Autodesk Fusion 360 part; units mm, degrees
box "BoxPrimitive5" add length 100 width 90 height 2 placed x (0, 0, -1) y (-1, 0, 0) z (0, 1, 0) at (0, 0, 0)
box "BoxPrimitive6" cut length 9 width 4 height -14 placed x (0, 0, 1) y (1, 0, 0) z (0, 1, 0) at (-6, 2, -9)
box "BoxPrimitive7" cut length 9 width 9 height -11 placed x (0, 0, -1) y (-1, 0, 0) z (0, 1, 0) at (-47, 2, -15)
box "BoxPrimitive8" cut length 9 width 9 height -10 placed x (0, 0, -1) y (-1, 0, 0) z (0, 1, 0) at (-47, 2, -76)
Input: part model. Units: mm. Frame: model coordinates. Round coordinates to 2 decimals unless told otherwise and drop trailing zeros. Loops run counter-clockwise (first coordinate to the right, second up) from the corner with the lowest first, then second, coordinate; pieces in that order, holes last. Notation, with made-up numbers: (39, -9.75) -> (93, -9.75) arc R31 cw to (93, 29.25) -> close; hole circle Ø8 at (56.5, -26). An arc over 180 degrees is marked (long way). Answer as a JSON object with one key per item and string values. Group by question number.
1) Ray query, L1, parallel to Z at x = -52, y = 0.75; L2, parallel to X at y = 0.65, z = -80.5. Return the intervals inside material, ascending.
2) Section query A-A on x = -52.5. Output: boundary loops of the cut face in (y, z), plus the area to 3 significant figures.
3) Section query B-B on y = 1.35. Output: boundary loops of the cut face in (x, z).
4) Pin query (flat end, axial travel): pin 1 (5 mm diameter, centred on x = -29.5, z = -66, fed in from -Y). Return the tip coordinate at first contact, or that it passes through.
Reply:
{
 "1": {"L1": "z = -100 to -85, -76 to -24, -15 to 0", "L2": "x = -90 to -56, -47 to 0"},
 "2": {"outline": "(0, -100) -> (2, -100) -> (2, -85) -> (0, -85) -> close; (0, -76) -> (2, -76) -> (2, -24) -> (0, -24) -> close; (0, -15) -> (2, -15) -> (2, 0) -> (0, 0) -> close", "area": "164 mm2"},
 "3": {"outline": "(-90, -100) -> (0, -100) -> (0, 0) -> (-2, 0) -> (-2, -9) -> (-6, -9) -> (-6, 0) -> (-90, 0) -> close; hole (-56, -85) -> (-47, -85) -> (-47, -76) -> (-56, -76) -> close; hole (-56, -24) -> (-47, -24) -> (-47, -15) -> (-56, -15) -> close"},
 "4": {"pin 1": "stops at y = 0"}
}
